Geometry: final body of the model. Coordinates: model frame, mm. A direction names the side the tool comes from. Coordinates: 2 decimals unless noted, no trailing zeros. Loops run counter-clockwise (first coordinate to the right, second up) from the corner with the lowest first, then second, coordinate; pieces in that order, holes last. Notation, with made-up numbers: (33, 68.25) - (79, 68.25) arc R19 cw to (79, 97.25) - close; hole circle Ø1 at (56, 19). An arc over 180 degrees is marked (long way). Return JSON: item names as keys, results as strings.
from build123d import *

# Parameters (mm, degrees)
F1_DEPTH = 38.1


with BuildPart() as f1:
    # F0 (on Front) → F1 (new body)
    with BuildSketch(Plane.XZ):
        Polygon((-35.56, 25.4), (-63.5, 25.4), (-58.603186, 17.78), (-40.54516, 17.78), align=None)
        Polygon((-2.54, 25.4), (-30.48, 25.4), (-25.583186, 17.78), (-7.52516, 17.78), align=None)
        Polygon((30.48, 25.4), (2.54, 25.4), (7.436814, 17.78), (25.49484, 17.78), align=None)
        Polygon((58.51484, 17.78), (63.5, 25.4), (35.56, 25.4), (40.456814, 17.78), align=None)
        Polygon((-63.5, 27.284326), (-63.5, 25.4), (-35.56, 25.4), (-30.48, 25.4), (-2.54, 25.4), (2.54, 25.4), (30.48, 25.4), (35.56, 25.4), (63.5, 25.4), (63.483231, 27.284326), align=None)
    extrude(amount=F1_DEPTH)


solid = f1.part
Item 1: Section query B-B, the plane y = -23.5. Return loops of the section in (x, z), and give its area (3 significant figures).
Worked out:
{"outline": "(-63.5, 25.4) - (-58.6, 17.78) - (-40.55, 17.78) - (-35.56, 25.4) - (-30.48, 25.4) - (-25.58, 17.78) - (-7.53, 17.78) - (-2.54, 25.4) - (2.54, 25.4) - (7.44, 17.78) - (25.49, 17.78) - (30.48, 25.4) - (35.56, 25.4) - (40.46, 17.78) - (58.51, 17.78) - (63.5, 25.4) - (63.48, 27.28) - (-63.5, 27.28) - close", "area": "940 mm^2"}
Item 2: Reachability of faces 1 (the face through (38, -18.8, 21.6)), 2 (the face through (-17, -19, 17.78)) from +Z, -Z, +X, -X, +Y, -Y: full face, straight path, thin tool, end or side. Return the list, or none.
Worked out:
{"face 1": "-Z, +Y, -Y", "face 2": "-Z, +X, -X, +Y, -Y"}
Item 3: First-contact query: pin 1 Ø4 at (x, y) = (1, -27) entering from -Z; pin 2 Ø5.5 at (x, y) = (-32.5, -21) entering from -Z; pin 3 Ø4 at (x, y) = (33, -28.5) entering from -Z. Flat tips, straight axial feed; report the tip coordinate or a pass-through.
Worked out:
{"pin 1": "z = 24.68", "pin 2": "z = 24.26", "pin 3": "z = 25.4"}
Item 4: Mould query, pull axis X, two halves, no side actions, for faces 3 (the face through (16, -19, 17.78)), 4 (the face through (-61.086, -18.783, 21.643)), 5 (the face through (-38.087, -18.783, 21.537)), 6 (the face through (60.973, -18.783, 21.537)). Classes: +X half, -X half, draft (parallel to the pull), parting line (faces both ways), or undercut.
Worked out:
{"face 3": "draft", "face 4": "-X half", "face 5": "undercut", "face 6": "+X half"}
Item 5: Section query A-A, the plane z = 22.5. Return loops of the section in (x, y).
Worked out:
{"outline": "(-61.64, -38.1) - (-37.46, -38.1) - (-37.46, 0) - (-61.64, 0) - close; (-28.62, -38.1) - (-4.44, -38.1) - (-4.44, 0) - (-28.62, 0) - close; (4.4, -38.1) - (28.58, -38.1) - (28.58, 0) - (4.4, 0) - close; (37.42, -38.1) - (61.6, -38.1) - (61.6, 0) - (37.42, 0) - close"}
Item 6: Section query C-C, the plane x = -34. Return loops of the section in (y, z), and give its area (3 significant figures).
Worked out:
{"outline": "(-38.1, 25.4) - (0, 25.4) - (0, 27.28) - (-38.1, 27.28) - close", "area": "71.8 mm^2"}
Item 7: Section query D-D, the plane x = 37. Return loops of the section in (y, z), and give its area (3 significant figures).
Worked out:
{"outline": "(-38.1, 23.16) - (0, 23.16) - (0, 27.28) - (-38.1, 27.28) - close", "area": "157 mm^2"}
Item 8: Ray query, probe 1 along X at (y, z) = (-34.5, 19); probe 2 along X at (y, z) = (-33.5, 25); probe 3 along Z at (x, y) = (-34, -15). Return the intervals inside material, ascending. Write a range as from..to.
Worked out:
{"probe 1": "-59.39..-39.75, -26.37..-6.73, 6.65..26.29, 39.67..59.31", "probe 2": "-63.24..-35.82, -30.22..-2.8, 2.8..30.22, 35.82..63.24", "probe 3": "25.4..27.28"}
